Read the model definition and answer for the solid it produces. Units are mm, in the model's axes. A direction names the side the tool comes from. Round coordinates to 2 decimals unless told otherwise and drop trailing zeros. Loops run counter-clockwise (first coordinate to the right, second up) from the corner with the lowest first, then second, coordinate; pieces in that order, holes last. Notation, with made-up numbers: (-19, 10) - (36, 10) arc R16 cw to (36, 16) - close; hole circle Ø2 at (35, 80.25). An arc over 180 degrees is marked (long way). Answer as CSV lines item,"result".
```python
from build123d import *

# Parameters (mm, degrees)
F0_W     = 32
F0_H     = 3.1
F1_DEPTH = 100
F2_DEPTH = 90


with BuildPart() as f1:
    # F0 (on Right) → F1 (new body)
    with BuildSketch(Plane.YZ):
        Polygon((-24.5385469525, 0), (0, 0), (29.0492966146, 0), (29.0492966146, 3.9169512209), (21.6441504219, 3.9169512209), (21.6441504219, 10.9582875453), (-18.4965940373, 10.9582875453), (-18.4965940373, 3.9169512209), (-24.5385469525, 3.9169512209), align=None)
        with Locations((1.6276613058, 5.4589794578)):
            Rectangle(F0_W, F0_H, mode=Mode.SUBTRACT)
        with Locations((1.6276613058, 5.4589794578)):
            Rectangle(F0_W, F0_H)
    extrude(amount=F1_DEPTH)

    # F0 (on Right) → F2 (cut, through all)
    with BuildSketch(Plane.YZ):
        with Locations((1.6276613058, 5.4589794578)):
            Rectangle(F0_W, F0_H)
    extrude(amount=F2_DEPTH, mode=Mode.SUBTRACT)


solid = f1.part
```
1) A cutting plane is placed at A-A, the plane x = 28. Determine the outline of the cut face in (y, z), plus the area to 3 significant figures.
Entries:
outline,"(-24.54, 0) - (29.05, 0) - (29.05, 3.92) - (21.64, 3.92) - (21.64, 10.96) - (-18.5, 10.96) - (-18.5, 3.92) - (-24.54, 3.92) - close; hole (-14.37, 3.91) - (17.63, 3.91) - (17.63, 7.01) - (-14.37, 7.01) - close"
area,"393 mm^2"
2) A cutting plane is placed at B-B, the plane y = 8. Determine the outline of the cut face in (x, z).
Entries:
outline,"(0, 0) - (100, 0) - (100, 10.96) - (0, 10.96) - (0, 7.01) - (90, 7.01) - (90, 3.91) - (0, 3.91) - close"
3) Find the intervals of material crossed by line 1 (Z direction, x = 73, y = 10.5); line 2 (Y direction, x = 8.5, z = 5.5); line 3 (Y direction, x = 15.5, z = 10), in increasing order.
Entries:
line 1,"z = 0 to 3.91, 7.01 to 10.96"
line 2,"y = -18.5 to -14.37, 17.63 to 21.64"
line 3,"y = -18.5 to 21.64"
4) Each of these flat-tipped pins is pushed along its axis until it touches: P1, Ø5, axis at x = 51, z = 6.5, coming from the +Y side; P2, Ø3.5, axis at x = 55, z = 6, coming from the -Y side; P3, Ø8, axis at x = 59.5, y = 26, coming from the +Z side. Where does it stop, or does it pass through?
Entries:
P1,"stops at y = 21.64"
P2,"stops at y = -18.5"
P3,"stops at z = 3.92"
5) The mould has two halves that part along Z. Classify faces 4 (the face through (44, 1, 3.909)), 5 (the face through (49, 25, 3.917)), 6 (the face through (44, 17.628, 5)), 7 (the face through (49, -24.539, 2)): pulls with the +Z half, pulls with the -Z half, needs draft (parallel to the pull), parting line crosses it, or undercut.
Entries:
face 4,"undercut"
face 5,"pulls with the +Z half"
face 6,"undercut"
face 7,"needs draft"
6) A cutting plane is placed at C-C, the plane z = 9.5. Determine the outline of the cut face in (x, y).
Entries:
outline,"(0, -18.5) - (100, -18.5) - (100, 21.64) - (0, 21.64) - close"
7) A tool of negligible diameter and unlimited length cuts with its end or side. For faces 1 (the face through (49, 21.644, 7)), 2 (the face through (44, -14.372, 5)), 3 (the face through (49, -21, 3.917)), from which of +Z, -Z, +X, -X, +Y, -Y can it reach the whole face along a straight path? Write none if from no direction.
Entries:
face 1,"+Z, +X, -X, +Y"
face 2,"-X"
face 3,"+Z, +X, -X, -Y"
